```python
from build123d import *

# Parameters (mm, degrees)
SKETCH1_R           = 7
BOSS_EXTRUDE1_DEPTH = 2
SKETCH2_R           = 4.95
BOSS_EXTRUDE2_DEPTH = 10
SKETCH3_R           = 2.6
CUT_EXTRUDE1_DEPTH  = 13
FILLET1_R           = 1


with BuildPart() as part:
    # Sketch1 → Boss-Extrude1 (new body)
    with BuildSketch(Plane(origin=(0, 0, 0), x_dir=(1, 0, 0), z_dir=(0, 1, 0))):
        Circle(SKETCH1_R)
    extrude(amount=BOSS_EXTRUDE1_DEPTH)

    # Sketch2 → Boss-Extrude2 (add)
    with BuildSketch(Plane(origin=(0, 2, 0), x_dir=(1, 0, 0), z_dir=(0, 1, 0))):
        Circle(SKETCH2_R)
    extrude(amount=BOSS_EXTRUDE2_DEPTH)

    # Sketch3 → Cut-Extrude1 (cut, through all)
    with BuildSketch(Plane.XZ):
        Circle(SKETCH3_R)
    extrude(amount=-CUT_EXTRUDE1_DEPTH, mode=Mode.SUBTRACT)

    # Fillet1
    fillet1_edges = [part.edges().sort_by_distance(p)[0] for p in [
        (-4.95, 12, 0),
    ]]
    fillet(fillet1_edges, radius=FILLET1_R)


solid = part.part
```
Can you work these out from the model? Positions are in its coordinate system, mm. A direction names the side the tool comes from. Coordinates: 2 decimals unless noted, no trailing zeros. Loops run counter-clockwise (first coordinate to the right, second up) from the corner with the lowest first, then second, coordinate; pieces in that order, holes last. Notation, with made-up numbers: (77, 18.25) - (127, 18.25) arc R28 cw to (127, 36.25) - close; hole circle Ø8 at (88.5, 51). An arc over 180 degrees is marked (long way). Use a Markdown table: item, result.
Item 1: I want a section at D-D on y = 1. Please give me the cut outline in (x, z).
Numbers:
| item | result |
|---|---|
| outline | circle Ø14 at (0, 0); hole circle Ø5.2 at (0, 0) |
Item 2: I want a section at A-A on z = 0. Please give me the cut outline in (x, y).
Numbers:
| item | result |
|---|---|
| outline | (-7, 0) - (-2.6, 0) - (-2.6, 12) - (-3.95, 12) arc R1 ccw to (-4.95, 11) - (-4.95, 2) - (-7, 2) - close; (2.6, 0) - (7, 0) - (7, 2) - (4.95, 2) - (4.95, 11) arc R1 ccw to (3.95, 12) - (2.6, 12) - close |
Item 3: I want a section at C-C on y = 10.75. Please give me the cut outline in (x, z), and give its area (3 significant figures).
Numbers:
| item | result |
|---|---|
| outline | circle Ø9.9 at (0, 0); hole circle Ø5.2 at (0, 0) |
| area | 55.7 mm2 |
Item 4: If I drill on probe 1 along Z at (x, y) = (0, 5); probe 2 along Y at (x, z) = (4, -0.25); probe 3 along Y at (x, z) = (6, -3), over which ranges is the centre line in solid material (lowest first)? Write a range as from..to.
Numbers:
| item | result |
|---|---|
| probe 1 | z = -4.95..-2.6, 2.6..4.95 |
| probe 2 | y = 0..12 |
| probe 3 | y = 0..2 |
Item 5: We'd pull the mould along Y, two halves only. Please class faces 3 (the face through (-0.338, 5.916, 2.578)), 4 (the face through (3, 12, 1)), 5 (the face through (0, 0, 3)): released by +Y, released by -Y, zero draft, split by the parting line, or undercut.
Numbers:
| item | result |
|---|---|
| face 3 | zero draft |
| face 4 | released by +Y |
| face 5 | released by -Y |
Item 6: For faces 1 (the face through (6.466, 0.986, 2.681)), 2 (the face through (4.72, 6.44, -1.49)), which set-ups out of +Z, -Z, +X, -X, +Y, -Y let a thin tool reach every point of the face, with its end or its side?
Numbers:
| item | result |
|---|---|
| face 1 | +Y, -Y |
| face 2 | +Y |
Item 7: I want a section at B-B on x = 0. Please give me the cut outline in (y, z).
Numbers:
| item | result |
|---|---|
| outline | (0, -7) - (2, -7) - (2, -4.95) - (11, -4.95) arc R1 ccw to (12, -3.95) - (12, -2.6) - (0, -2.6) - close; (0, 2.6) - (12, 2.6) - (12, 3.95) arc R1 ccw to (11, 4.95) - (2, 4.95) - (2, 7) - (0, 7) - close |
Item 8: Will these pins go through, and if not, where does the flat tip stop? pin 1 (3 mm diameter, centred on y = 8.5, z = -2.5, fed in from +X); pin 2 (2 mm diameter, centred on x = -1, y = 6, fed in from -Z).
Numbers:
| item | result |
|---|---|
| pin 1 | stops at x = 4.85 |
| pin 2 | stops at z = -4.95 |
